Autodesk Inventor part; units mm, degrees
ref_plane "YZ Plane" through (0, 0, 0) normal (1, 0, 0) x (0, 1, 0)
ref_plane "XZ Plane" through (0, 0, 0) normal (0, 1, 0) x (-1, 0, 0)
ref_plane "XY Plane" through (0, 0, 0) normal (0, 0, 1) x (1, 0, 0)
sketch "Skizze_Grundkörper" plane through (0, 0, 0) normal (0, 0, 1) x (1, 0, 0)
  line L0 (-56, 0) -> (56, 0)
  line L1 (0, -45.5) -> (0, 45.5)
  line L2 (35, -30) -> (-35, -30)
  line L3 (-35, -30) -> (-35, 30)
  line L4 (-35, 30) -> (35, 30)
  line L5 (35, 30) -> (35, -30)
  line L6 (35, -30) -> (-35, 30) construction
  line L7 (-35, -30) -> (35, 30) construction
  point P0 (0, 0)
  dimension "Länge" = 70
  dimension "Höhe" = 60
extrude "Grundkörper" add sketch "Skizze_Grundkörper" along normal blind 10
sketch "Skizze2" plane through (0, 0, 10) normal (0, 0, 1) x (1, 0, 0)
  line L0 (-35, -30) -> (35, -30)
  line L1 (35, -30) -> (35, 30)
  line L2 (35, 30) -> (-35, 30)
  line L3 (-35, 30) -> (-35, -30)
  line L4 (-56, 0) -> (56, 0)
  line L5 (0, -45.5) -> (0, 45.5)
  point P0 (0, 0)
  point P1 (0, 18)
  dimension "d4" = 48
hole "Bohrung_9,7_mm" at (0, 18, 10) direction (0, 0, -1) diameter 9.7 end through all
sketch "Skizze3" plane through (0, 0, 10) normal (0, 0, 1) x (1, 0, 0)
  circle A0 centre (0, 18) radius 4.85
  line L0 (-35, -30) -> (35, -30)
  line L1 (35, -30) -> (35, 30)
  line L2 (35, 30) -> (-35, 30)
  line L3 (-35, 30) -> (-35, -30)
  line L4 (-56, 0) -> (56, 0)
  line L5 (0, -45.5) -> (0, 45.5)
  point P0 (0, 0)
  point P1 (-25, -24)
  point P2 (25, -24)
  dimension "d12" = 50
  dimension "d13" = 6
hole "Bohrung_5,5_mm" at (-25, -24, 10) at (25, -24, 10) direction (0, 0, -1) diameter 5.5 end through all
chamfer "Fase_10_mm" distance 10 angle 45 2 edges at (-35, 30, 5) (35, 30, 5)
properties material "Stahl, unlegiert"
Source: CAD feature listing. Evaluate the final solid. Frame: model axes, mm. Round coordinates to 2 decimals unless told otherwise and drop trailing zeros. Loops run counter-clockwise (first coordinate to the right, second up) from the corner with the lowest first, then second, coordinate; pieces in that order, holes last. Notation, with made-up numbers: M 45.25,39.25 L 68.25,39.25 A28 cw 68.25,70.25 Z; hole C 71.25,46.5 d2. An arc over 180 degrees is marked long. Use a Markdown table: item, result. Add a question column.
1. Cut plane C-C, the plane x = 3.5. Output: boundary loops of the cut face in (y, z), and give its area (3 significant figures).
2. Ray query, line 1 along X through (y, z) = (-24, 4.5); line 2 along Y through (x, z) = (0, 3.75); line 3 along X through (y, z) = (18, 4.5). Return the intervals inside material, ascending. Write a range as [from, to].
3. Cut plane D-D, the plane y = 25. Output: boundary loops of the cut face in (x, z), and give its area (3 significant figures).
4. Pull-direction query (Y, two-part tool) for faces 1 (the cylindrical face through (-0.213, 22.845, 4.93)), 2 (the flat face through (0, 0, 0)), 3 (the flat face through (30, 25, 5)); classes: +Y half, -Y half, draft (parallel to the pull), parting line (faces both ways), or undercut.
5. Cut plane A-A, the plane z = 1. Output: boundary loops of the cut face in (x, y).
6. Cut plane B-B, the plane y = -24. Output: boundary loops of the cut face in (x, z), and give its area (3 significant figures).
7. Contact query for flat-ended pins moving along their axis: pin 1 (1 mm diameter, centred on y = 21, z = 7, fed in from -X); pin 2 (1 mm diameter, centred on x = 27, z = 8.5, fed in from +Y). Output: stop coordinate, or through.
Solution:
| question | item | result |
|---|---|---|
| 1 | outline | M -30,0 L 14.64,0 L 14.64,10 L -30,10 Z; M 21.36,0 L 30,0 L 30,10 L 21.36,10 Z |
| 1 | area | 533 mm2 |
| 2 | line 1 | x = [-35, -27.75], [-22.25, 22.25], [27.75, 35] |
| 2 | line 2 | y = [-30, 13.15], [22.85, 30] |
| 2 | line 3 | x = [-35, -4.85], [4.85, 35] |
| 3 | outline | M -30,0 L 30,0 L 30,10 L -30,10 Z |
| 3 | area | 600 mm2 |
| 4 | face 1 | undercut |
| 4 | face 2 | draft |
| 4 | face 3 | +Y half |
| 5 | outline | M -35,-30 L 35,-30 L 35,20 L 25,30 L -25,30 L -35,20 Z; hole C -25,-24 d5.5; hole C 0,18 d9.7; hole C 25,-24 d5.5 |
| 6 | outline | M -35,0 L -27.75,0 L -27.75,10 L -35,10 Z; M -22.25,0 L 22.25,0 L 22.25,10 L -22.25,10 Z; M 27.75,0 L 35,0 L 35,10 L 27.75,10 Z |
| 6 | area | 590 mm2 |
| 7 | pin 1 | stops at x = -34.5 |
| 7 | pin 2 | stops at y = 28.5 |
